```python
from build123d import *

# Parameters (mm, degrees)
SKETCH1_R           = 5
BOSS_EXTRUDE1_DEPTH = 20
SKETCH3_R           = 2.5
BOSS_EXTRUDE2_DEPTH = 40
SKETCH7_R           = 1.5
CUT_EXTRUDE1_DEPTH  = 62.032778079
SKETCH9_R           = 1.5
CUT_EXTRUDE2_DEPTH  = 121.519707944


with BuildPart() as part:
    # Sketch1 → Boss-Extrude1 (new body)
    with BuildSketch(Plane.XY):
        Circle(SKETCH1_R)
    boss_extrude1 = extrude(amount=BOSS_EXTRUDE1_DEPTH)

    # Sketch3 → Boss-Extrude2 (add)
    with BuildSketch(Plane.XY.offset(20)):
        Circle(SKETCH3_R)
    boss_extrude2 = extrude(amount=BOSS_EXTRUDE2_DEPTH)

    # Sketch7 → Cut-Extrude1 (cut, through all)
    with BuildSketch(Plane(origin=(5, 0, 0), x_dir=(0, 0, -1), z_dir=(1, 0, 0))):
        with Locations((-5, 0)):
            Circle(SKETCH7_R)
    extrude(amount=-CUT_EXTRUDE1_DEPTH, mode=Mode.SUBTRACT)

    # Mirror4: Boss-Extrude2 across plane
    add(boss_extrude2.mirror(Plane.XY.offset(60)))

    # Mirror5: Boss-Extrude1 across plane
    add(boss_extrude1.mirror(Plane.XY.offset(60)))

    # Sketch9 → Cut-Extrude2 (cut, through all)
    with BuildSketch(Plane(origin=(5, 0, 0), x_dir=(0, 0, -1), z_dir=(1, 0, 0))):
        with Locations((-115, 0)):
            Circle(SKETCH9_R)
    extrude(amount=-CUT_EXTRUDE2_DEPTH, mode=Mode.SUBTRACT)


solid = part.part
```
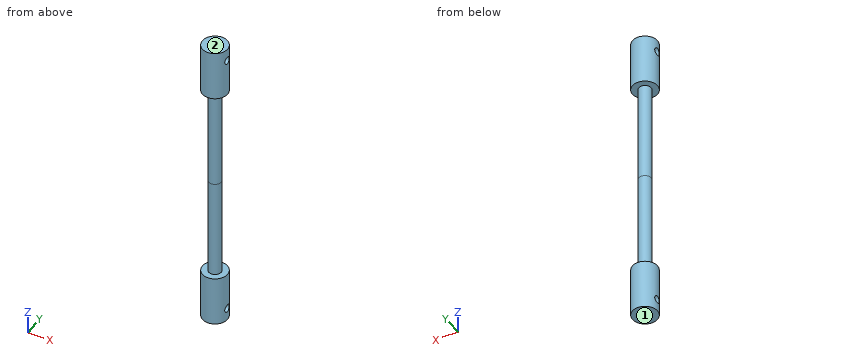
Can you work these out from the model? Positions are in its coordinate system, mm. Face numbers are marked on the shaded views. Give positions to 0.01 mm unless a question says otherwise; leave off trailing zeros. Order: outer loops, then holes, each group sorted by start corner. A loop starts at its lowest first (then second) coordinate and runs counter-clockwise, first axis right, second up. Notation, with made-up numbers: (-11, -15.5) - (27, -15.5) arc R29 cw to (27, 17.5) - close; hole circle Ø8 at (-3, 83). An arc over 180 degrees is marked (long way). Use a Markdown table: item, result. Add a question column.
Q1. If we section it at C-C on z = 115: Write out the boundary of the cut face in (x, y).
Q2. If we mould it in two halves opening along Z, with no side actions, what happens to the marked faces 1 and 2? For each: released by +Z, released by -Z, zero draft, split by the parting line, or undercut.
Q3. If we section it at B-B on z = 63: Write out the boundary of the cut face in (x, y), plus the area to 3 significant figures.
Q4. If we section it at A-A on x = 3.5: Write out the boundary of the cut face in (y, z), plus the area to 3 significant figures.
Q5. Please list where these lines run through material, in increasing order: line 1 along Z through (x, y) = (2.25, 0); line 2 along Z through (x, y) = (3, 0); line 3 along Z through (x, y) = (-2.5, 3.5).
Q6. I'm going to push flat-ended pins straight in: pin 1 (1 mm diameter, centred on x = -3, z = 13.5, fed in from -Y); pin 2 (2.5 mm diameter, centred on y = 0, z = 115, fed in from +X); pin 3 (2 mm diameter, centred on y = 1.5, z = 94.5, fed in from +X); pin 4 (1 mm diameter, centred on x = 0.5, z = 25, fed in from -Y). Where does each tip first touch, or does it pass through?
Answers follow:
| question | item | result |
|---|---|---|
| 1 | outline | (-4.77, -1.5) arc R5 ccw to (4.77, -1.5) - close; (-4.77, 1.5) - (4.77, 1.5) arc R5 ccw to start |
| 2 | face 1 | released by -Z |
| 2 | face 2 | released by +Z |
| 3 | outline | circle Ø5 at (0, 0) |
| 3 | area | 19.6 mm^2 |
| 4 | outline | (-3.57, 0) - (3.57, 0) - (3.57, 20) - (-3.57, 20) - close; (-3.57, 100) - (3.57, 100) - (3.57, 120) - (-3.57, 120) - close; hole circle Ø3 at (0, 5); hole circle Ø3 at (0, 115) |
| 4 | area | 272 mm^2 |
| 5 | line 1 | z = 0 to 3.5, 6.5 to 113.5, 116.5 to 120 |
| 5 | line 2 | z = 0 to 3.5, 6.5 to 20, 100 to 113.5, 116.5 to 120 |
| 5 | line 3 | z = 0 to 20, 100 to 120 |
| 6 | pin 1 | stops at y = -4.33 |
| 6 | pin 2 | passes through |
| 6 | pin 3 | stops at x = 2.45 |
| 6 | pin 4 | stops at y = -2.5 |
